from build123d import *

# Parameters (mm, degrees)
SKETCH1_W           = 10
SKETCH1_H           = 5
BOSS_EXTRUDE1_DEPTH = 2.5
CUT_EXTRUDE2_REACH  = 141.432
SKETCH2_W           = 5
SKETCH2_H           = 5


with BuildPart() as part:
    # Sketch1 → Boss-Extrude1 (new, symmetric)
    with BuildSketch(Plane(origin=(0, 0, 0), x_dir=(-1, 0, 0), z_dir=(0, 1, 0))):
        with BuildLine():
            ThreePointArc((138.434966494, 10.875), (135.24177294, 5.848962219), (134.125, 0))
            Line((134.125, 0), (-134.125, 0))
            ThreePointArc((-134.125, 0), (-135.24177294, 5.848962219), (-138.434966494, 10.875))
            Line((-138.434966494, 10.875), (138.434966494, 10.875))
        make_face()
        with Locations((-77.04, 13.375)):
            Rectangle(SKETCH1_W, SKETCH1_H)
        with Locations((77.04, 13.375)):
            Rectangle(SKETCH1_W, SKETCH1_H)
    extrude(amount=BOSS_EXTRUDE1_DEPTH, both=True)

    # Sketch2 → Cut-Extrude2 (cut, up to next)
    with BuildSketch(Plane(origin=(0, 2.5, 0), x_dir=(-1, 0, 0), z_dir=(0, 1, 0)), mode=Mode.PRIVATE) as cut_extrude2_sk1:
        with Locations((-11.455033506, 8.375)):
            Rectangle(SKETCH2_W, SKETCH2_H)
    cut_extrude2_tool1 = extrude(cut_extrude2_sk1.sketch, amount=-CUT_EXTRUDE2_REACH, mode=Mode.PRIVATE) & part.part
    # Sketch2 → Cut-Extrude2 (cut, up to next)
    with BuildSketch(Plane(origin=(0, 2.5, 0), x_dir=(-1, 0, 0), z_dir=(0, 1, 0)), mode=Mode.PRIVATE) as cut_extrude2_sk2:
        with Locations((15.544966494, 8.375)):
            Rectangle(SKETCH2_W, SKETCH2_H)
    cut_extrude2_tool2 = extrude(cut_extrude2_sk2.sketch, amount=-CUT_EXTRUDE2_REACH, mode=Mode.PRIVATE) & part.part
    add(cut_extrude2_tool1.solids().sort_by_distance((11.455034, 2.5, 8.375))[0], mode=Mode.SUBTRACT)
    add(cut_extrude2_tool2.solids().sort_by_distance((-15.544966, 2.5, 8.375))[0], mode=Mode.SUBTRACT)


solid = part.part
Geometry check sheet. Reference: the model listing, model coordinates, mm. A direction names the side the tool comes from. Coordinates: 2 decimals unless noted, no trailing zeros. Order: outer loops, then holes, each group sorted by start corner. A loop starts at its lowest first (then second) coordinate and runs counter-clockwise, first axis right, second up. Notation, with made-up numbers: (-34.75, 67.5) - (-2.75, 67.5) arc R8 ccw to (-2.75, 79.5) - close; hole circle Ø3 at (-21, 49). An arc over 180 degrees is marked (long way). Answer in a Markdown table with one row per item. Add a question column.
1) Cross-section at A-A, the plane y = -0.4. Record the cut outline in (x, z) (3 decimals), then the cut area to 3 significant figures.
2) Release check for a two-part mould opening along X. For faces 1 (the cylindrical face through (135.21, 0.04, 5.77)), 2 (the flat face through (-16, 0, 5.875)), 3 (the flat face through (-110, 0, 10.875)) record: +X half, -X half, draft (parallel to the pull), parting line (faces both ways), or undercut.
3) Gauge pin test, flat ends, axial feed: P1, Ø2.5, axis at x = -15, y = -0.5, coming from the +Z side (3 decimals); P2, Ø1.5, axis at y = 0, z = 7.5, coming from the -X side; P3, Ø2.5, axis at x = -115.5, y = 1, coming from the +Z side (3 decimals). Record the tip position at first contact, or that the pin passes through.
4) Material ranges on line 1 along X through (y, z) = (0.35, 13); line 2 along X through (y, z) = (1.3, 10); line 3 along X through (y, z) = (2, 1), recorded low to high. Write a range as [from, to].
5) Set-up check for faces 4 (the flat face through (111, 0, 10.875)), 5 (the flat face through (-72.04, 0, 13)), 6 (the flat face through (-82.04, 0, 13)), 7 (the flat face through (-77, 0, 15.875)): record each of +Z, -Z, +X, -X, +Y, -Y from which the full face is reachable in a straight line by a thin tool's end or side.
6) Cross-section at B-B, the plane x = -32.5. Record the cut outline in (y, z) (3 decimals).
Check result:
| question | item | result |
|---|---|---|
| 1 | outline | (-138.435, 10.875) arc R15.875 cw to (-134.125, 0) - (134.125, 0) arc R15.875 cw to (138.435, 10.875) - (82.04, 10.875) - (82.04, 15.875) - (72.04, 15.875) - (72.04, 10.875) - (13.955, 10.875) - (13.955, 5.875) - (8.955, 5.875) - (8.955, 10.875) - (-13.045, 10.875) - (-13.045, 5.875) - (-18.045, 5.875) - (-18.045, 10.875) - (-72.04, 10.875) - (-72.04, 15.875) - (-82.04, 15.875) - (-82.04, 10.875) - close |
| 1 | area | 3,000 mm² |
| 2 | face 1 | +X half |
| 2 | face 2 | undercut |
| 2 | face 3 | draft |
| 3 | P1 | stops at z = 5.875 |
| 3 | P2 | stops at x = -136.44 |
| 3 | P3 | stops at z = 10.875 |
| 4 | line 1 | x = [-82.04, -72.04], [72.04, 82.04] |
| 4 | line 2 | x = [-137.67, -18.04], [-13.04, 8.96], [13.96, 137.67] |
| 4 | line 3 | x = [-134.16, 134.16] |
| 5 | face 4 | +Z, +X, +Y, -Y |
| 5 | face 5 | +Z, +Y, -Y |
| 5 | face 6 | +Z, -X, +Y, -Y |
| 5 | face 7 | +Z, +X, -X, +Y, -Y |
| 6 | outline | (-2.5, 0) - (2.5, 0) - (2.5, 10.875) - (-2.5, 10.875) - close |
